For this review, take the finished solid that the model builds, in its own axes (mm). Face numbers are marked on the shaded views. A direction names the side the tool comes from. Give positions to 0.01 mm unless a question says otherwise; leave off trailing zeros. Write each loop counter-clockwise with the first axis right and the second up, starting at its lowest first coordinate (ties: lowest second). Pieces come first, ordered by that corner, then holes. Notation, with made-up numbers: (67.25, 83) -> (89.25, 83) arc R23 cw to (89.25, 103) -> close; hole circle Ø5 at (87.5, 54). An arc over 180 degrees is marked (long way). Return JSON: item names as keys, results as strings.
from build123d import *
from OCP.BRepFilletAPI import BRepFilletAPI_MakeChamfer

# Parameters (mm, degrees)
SKETCH1_R               = 13
BOSS_EXTRUDE1_DEPTH     = 10
SKETCH3_R               = 17
BOSS_EXTRUDE2_DEPTH     = 2
F_4_MM_SHAFT_HOLE_DEPTH = 27.870057685
BOSS_EXTRUDE3_START     = 2
SKETCH9_R               = 17
SKETCH9_R_2             = 2.25
BOSS_EXTRUDE3_DEPTH     = 2
CUT_EXTRUDE3_DEPTH      = 27.038433133
CUT_EXTRUDE4_START      = 10
SKETCH10_3_R            = 2
SKETCH10_3_R_2          = 1.5
CUT_EXTRUDE4_DEPTH      = 17.038433171
CUT_EXTRUDE5_DEPTH      = 4
FILLET3_R               = 6
FILLET4_R               = 0.5
CHAMFER1_SIZE           = 1
CUT_EXTRUDE7_DEPTH      = 2
FILLET6_R               = 5
FILLET8_R               = 0.2
CHAMFER3_SIZE           = 1
CHAMFER3_SIZE2          = 0.531709432


with BuildPart() as part:
    # Sketch1 → Boss-Extrude1 (new body)
    with BuildSketch(Plane(origin=(0, 0, 0), x_dir=(1, 0, 0), z_dir=(0, 1, 0))):
        with Locations(Location((0, 0, 0), (0, 0, 270))):
            Circle(SKETCH1_R)
    extrude(amount=BOSS_EXTRUDE1_DEPTH)

    # Sketch2 → Cut-Revolve1 (revolve, cut)
    with BuildSketch(Plane(origin=(0, 0, 0), x_dir=(0, 0, -1), z_dir=(1, 0, 0)), mode=Mode.PRIVATE) as cut_revolve1_sk:
        Polygon((-13, 0), (-10.771428571, 10), (-13, 10), align=None)
    revolve(cut_revolve1_sk.sketch.rotate(Axis((0, 0, 0), (0, 1, 0)), 180), axis=Axis((0, 0, 0), (0, 1, 0)), mode=Mode.SUBTRACT)

    # Sketch3 → Boss-Extrude2 (add)
    with BuildSketch(Plane(origin=(0, 0, 0), x_dir=(-1, 0, 0), z_dir=(0, -1, 0))):
        with Locations(Location((0, 0, 0), (0, 0, 90))):
            Circle(SKETCH3_R)
    extrude(amount=BOSS_EXTRUDE2_DEPTH)

    # Sketch5 → 4-mm shaft hole (cut, through all)
    with BuildSketch(Plane(origin=(0, 10, 0), x_dir=(1, 0, 0), z_dir=(0, 1, 0))):
        with BuildLine():
            ThreePointArc((1.677050983, 1.5), (0, 2.25), (-1.677050983, 1.5))
            Line((-1.677050983, 1.5), (1.677050983, 1.5))
        make_face()
        with BuildLine():
            Line((1.677050983, 1.5), (-1.677050983, 1.5))
            ThreePointArc((-1.677050983, 1.5), (-0.802849702, -2.101887808), (2.25, 0))
            ThreePointArc((2.25, 0), (2.101887808, 0.802849702), (1.677050983, 1.5))
        make_face()
    extrude(amount=-F_4_MM_SHAFT_HOLE_DEPTH, mode=Mode.SUBTRACT)

    # Sketch9 → Boss-Extrude3 (add)
    with BuildSketch(Plane(origin=(0, 0, 0), x_dir=(1, 0, 0), z_dir=(0, 1, 0)).offset(BOSS_EXTRUDE3_START)):
        with Locations(Location((0, 0, 0), (0, 0, 270))):
            Circle(SKETCH9_R)
        with Locations(Location((0, 0, 0), (0, 0, 270))):
            Circle(SKETCH9_R_2, mode=Mode.SUBTRACT)
    extrude(amount=-BOSS_EXTRUDE3_DEPTH)

    # Sketch10 → Cut-Extrude3 (cut, through all)
    with BuildSketch(Plane.XY):
        with BuildLine():
            ThreePointArc((0, 7.5), (-1.5, 6), (0, 4.5))
            Line((0, 4.5), (0, 7.5))
        make_face()
        with BuildLine():
            Line((0, 7.5), (0, 4.5))
            ThreePointArc((0, 4.5), (1.060660172, 4.939339828), (1.5, 6))
            ThreePointArc((1.5, 6), (1.060660172, 7.060660172), (0, 7.5))
        make_face()
    extrude(amount=CUT_EXTRUDE3_DEPTH, mode=Mode.SUBTRACT)

    # Sketch10<3> → Cut-Extrude4 (cut, through all)
    with BuildSketch(Plane.XY.offset(CUT_EXTRUDE4_START)):
        with Locations(Location((0, 6, 0), (0, 0, 225.143578884))):
            Circle(SKETCH10_3_R)
        with Locations(Location((0, 6, 0), (0, 0, 270))):
            Circle(SKETCH10_3_R_2, mode=Mode.SUBTRACT)
    extrude(amount=CUT_EXTRUDE4_DEPTH, mode=Mode.SUBTRACT)

    # Sketch11 → Cut-Extrude5 (cut)
    with BuildSketch(Plane(origin=(0, 10, 0), x_dir=(1, 0, 0), z_dir=(0, 1, 0))):
        with BuildLine():
            ThreePointArc((3, -8.242448615), (7.185132041, -5.031087033), (8.771428571, 0))
            ThreePointArc((8.771428571, 0), (5.031087033, 7.185132041), (-3, 8.242448615))
            ThreePointArc((-3, 8.242448615), (-6.302331872, 0.944417603), (0, -4))
            ThreePointArc((0, -4), (-4, 0), (0, 4))
            ThreePointArc((0, 4), (6.302331872, -0.944417603), (3, -8.242448615))
        make_face()
    extrude(amount=-CUT_EXTRUDE5_DEPTH, mode=Mode.SUBTRACT)

    # Fillet3
    fillet3_edges = [part.edges().sort_by_distance(p)[0] for p in [
        (-3, 8, -8.242448615),
    ]]
    fillet(fillet3_edges, radius=FILLET3_R)

    # Fillet4
    # the kernel refuses this fillet: 0.5 mm, written as the material it adds along each edge
    with BuildSketch(Plane(origin=(3, 10, 8.242448615), x_dir=(0.676109910174844, 0, -0.7368007799692969), z_dir=(0, -1, 0))) as fillet4_piece_1_section:
        with BuildLine():
            CenterArc((4.592297125, 0.470079575), FILLET4_R, 86.204134404, 163.874166307)
            ThreePointArc((4.625398075, 0.968982699), (2.246212442, 0.801862309), (0, 0))
            ThreePointArc((0, 0), (2.210964653, 0.38829518), (4.421929307, 0))
        make_face()
    fillet4_piece_1 = extrude(amount=15.814513008, mode=Mode.PRIVATE)
    fillet4_piece_1 = split(fillet4_piece_1, bisect_by=Plane(origin=(5.361441464, -2, 6.517574012), z_dir=(0, 1, 0)), keep=Keep.TOP, mode=Mode.PRIVATE)
    add(fillet4_piece_1)
    with BuildSketch(Plane(origin=(0, 10, 4), x_dir=(-0.8427994583990877, 0, -0.5382277147473964), z_dir=(0, -1, 0))) as fillet4_piece_2_section:
        with BuildLine():
            CenterArc((4.574935575, -0.421399729), FILLET4_R, 122.563073018, 157.850467981)
            ThreePointArc((4.665311372, -0.913164119), (2.246019142, -0.899203979), (0, 0))
            ThreePointArc((0, 0), (2.152910859, -0.628802166), (4.305821718, 0))
        make_face()
    fillet4_piece_2 = extrude(amount=14.384601093, mode=Mode.PRIVATE)
    fillet4_piece_2 = fillet4_piece_2 - Plane(origin=(0, 6, 2.911656579), x_dir=(0, 1, 0), z_dir=(0, 0, -1)) * Cylinder(1.5, 48, mode=Mode.PRIVATE)
    fillet4_piece_2 = split(fillet4_piece_2, bisect_by=Plane(origin=(-3.011239117, -2, 2.911656579), z_dir=(0, 1, 0)), keep=Keep.TOP, mode=Mode.PRIVATE)
    add(fillet4_piece_2)

    # Chamfer1
    chamfer1_edges = [part.edges().sort_by_distance(p)[0] for p in [
        (-3.371197834, 10, -2.152910859),
        (5.398969594, 10, -1.110594427),
        (-3.768481471, 10, -7.717945042),
        (7.597652385, 10, -4.383336334),
        (-6.424305098, 10, -1.576218344),
        (6.196119079, 10, 5.606673983),
        (-3.789032474, 10, 2.297570227),
    ]]
    chamfer(chamfer1_edges, length=CHAMFER1_SIZE)

    # Sketch14 → Cut-Extrude7 (cut)
    with BuildSketch(Plane(origin=(0, 10, 0), x_dir=(1, 0, 0), z_dir=(0, 1, 0))):
        with BuildLine():
            ThreePointArc((3.108583846, -2.517281564), (-5.049231929, -4.075420571), (-7.949614017, 3.706965896))
            ThreePointArc((-7.949614017, 3.706965896), (-7.397747824, -4.712885136), (0, -8.771428571))
            ThreePointArc((0, -8.771428571), (3.750591207, -5.184029494), (4, 0))
            ThreePointArc((4, 0), (3.770565964, -1.335227437), (3.108583846, -2.517281564))
        make_face()
    extrude(amount=-CUT_EXTRUDE7_DEPTH, mode=Mode.SUBTRACT)

    # Fillet6
    fillet6_edges = [part.edges().sort_by_distance(p)[0] for p in [
        (0, 9, 8.771428571),
    ]]
    fillet(fillet6_edges, radius=FILLET6_R)

    # Fillet8
    fillet8_edges = [part.edges().sort_by_distance(p)[0] for p in [
        (4, 9, 0),
        (-7.949614017, 9, -3.706965896),
    ]]
    fillet(fillet8_edges, radius=FILLET8_R)

    # Chamfer3: one chamfer whose edges measure the first distance from different faces: ONE call of the kernel's chamfer builder (chamfer() names one face for all edges)
    chamfer3_edges_1 = [part.edges().sort_by_distance(p)[0] for p in [
        (3.573698882, 10, 1.796851775),
    ]]
    chamfer3_side_1 = [part.faces().sort_by_distance(p)[0] for p in [
        (3.573698882, 9, 1.796851775),
    ]]
    chamfer3_edges_2 = [part.edges().sort_by_distance(p)[0] for p in [
        (-3.810129446, 10, 4.610453161),
    ]]
    chamfer3_side_2 = [part.faces().sort_by_distance(p)[0] for p in [
        (-3.810129446, 9, 4.610453161),
    ]]
    chamfer3_edges_3 = [part.edges().sort_by_distance(p)[0] for p in [
        (0.233729709, 10, 8.415761951),
    ]]
    chamfer3_side_3 = [part.faces().sort_by_distance(p)[0] for p in [
        (0.233729709, 9, 8.415761951),
    ]]
    chamfer3_edges_4 = [part.edges().sort_by_distance(p)[0] for p in [
        (-7.362823163, 10, 4.767262763),
    ]]
    chamfer3_side_4 = [part.faces().sort_by_distance(p)[0] for p in [
        (-7.362823163, 9, 4.767262763),
    ]]
    chamfer3_edges_5 = [part.edges().sort_by_distance(p)[0] for p in [
        (4.128369515, 10, 4.145305416),
    ]]
    chamfer3_side_5 = [part.faces().sort_by_distance(p)[0] for p in [
        (4.128369515, 9, 4.145305416),
    ]]
    chamfer3_edges_6 = [part.edges().sort_by_distance(p)[0] for p in [
        (-8.504611001, 10, -1.231596345),
    ]]
    chamfer3_side_6 = [part.faces().sort_by_distance(p)[0] for p in [
        (-8.504611001, 9, -1.231596345),
    ]]
    chamfer3_edges_7 = [part.edges().sort_by_distance(p)[0] for p in [
        (4.075125782, 10, 0.843648275),
    ]]
    chamfer3_side_7 = [part.faces().sort_by_distance(p)[0] for p in [
        (4.075125783, 9, 0.843648274),
    ]]
    chamfer3 = BRepFilletAPI_MakeChamfer(part.part.solid().wrapped)
    for e in chamfer3_edges_1:
        chamfer3.Add(CHAMFER3_SIZE, CHAMFER3_SIZE2, e.wrapped, chamfer3_side_1[0].wrapped)  # the first distance lies on this face
    for e in chamfer3_edges_2:
        chamfer3.Add(CHAMFER3_SIZE, CHAMFER3_SIZE2, e.wrapped, chamfer3_side_2[0].wrapped)  # the first distance lies on this face
    for e in chamfer3_edges_3:
        chamfer3.Add(CHAMFER3_SIZE, CHAMFER3_SIZE2, e.wrapped, chamfer3_side_3[0].wrapped)  # the first distance lies on this face
    for e in chamfer3_edges_4:
        chamfer3.Add(CHAMFER3_SIZE, CHAMFER3_SIZE2, e.wrapped, chamfer3_side_4[0].wrapped)  # the first distance lies on this face
    for e in chamfer3_edges_5:
        chamfer3.Add(CHAMFER3_SIZE, CHAMFER3_SIZE2, e.wrapped, chamfer3_side_5[0].wrapped)  # the first distance lies on this face
    for e in chamfer3_edges_6:
        chamfer3.Add(CHAMFER3_SIZE, CHAMFER3_SIZE2, e.wrapped, chamfer3_side_6[0].wrapped)  # the first distance lies on this face
    for e in chamfer3_edges_7:
        chamfer3.Add(CHAMFER3_SIZE, CHAMFER3_SIZE2, e.wrapped, chamfer3_side_7[0].wrapped)  # the first distance lies on this face
    add(Compound.cast(chamfer3.Shape()), mode=Mode.REPLACE)


solid = part.part
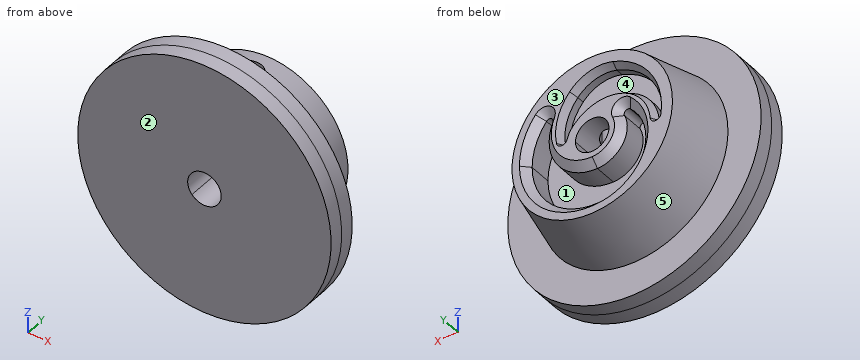
1. Add section A-A, the plane z = 14. State the section outline as (x, y) points.
Results found:
{"outline": "(-9.64, -2) -> (9.64, -2) -> (9.64, 2) -> (-9.64, 2) -> close"}
2. For the marked faces 1 and 2, list the 3-axis set-ups (+Z, -Z, +X, -X, +Y, -Y) from which the entire face can be reached by the end or side of a thin tool; tool diameter is ignored.
Results found:
{"face 1": "+Y", "face 2": "+Z, -Z, +X, -X, -Y"}
3. For pin 1 (1.5 mm diameter, centred on y = 3.5, z = 10.5, fed in from -X); pin 2 (11.5 mm diameter, centred on x = 2, z = -0.5, fed in from +Y); pin 3 (1.2 mm diameter, centred on x = -0.5, y = 6, fed in from +Z); pin 4 (1 mm diameter, centred on x = 2, y = 2, fed in from -Z), all flat-tipped, find the tip position at first contact; note any pin that passes through.
Results found:
{"pin 1": "stops at x = -7.4", "pin 2": "stops at y = 10", "pin 3": "stops at z = -1.96", "pin 4": "stops at z = -16.93"}
4. The part is to be moulded in two halves that separate along X. For the marked faces 3, 4 and 5, say which applies: +X half, -X half, draft (parallel to the pull), parting line (faces both ways), or undercut.
Results found:
{"face 3": "draft", "face 4": "undercut", "face 5": "parting line"}
5. To check wall thickness, follow probe 1 along Y at (x, z) = (13.5, -9.5); probe 2 along Y at (x, z) = (-5.5, 4); probe 3 along Z at (x, y) = (0, 1). State the ranges of each line that lie inside material, in increasing order.
Results found:
{"probe 1": "y = -2 to 2", "probe 2": "y = -2 to 8", "probe 3": "z = -17 to -2.25, 2.25 to 17"}
